Geometry: final body of the model. Coordinates: model frame, mm. A direction names the side the tool comes from. Coordinates: 2 decimals unless noted, no trailing zeros. Loops run counter-clockwise (first coordinate to the right, second up) from the corner with the lowest first, then second, coordinate; pieces in that order, holes last. Notation, with made-up numbers: (10, -34.75) - (43, -34.75) arc R18 cw to (43, -20.75) - close; hole circle Ø5 at (-32.5, 52). An arc over 180 degrees is marked (long way). Answer in a Markdown table with one row per item.
from build123d import *

# Parameters (mm, degrees)
SKETCH_R        = 14
SKETCH_R_2      = 2.5
PAD_DEPTH       = 16
SKETCH001_R     = 9
SKETCH001_R_2   = 2.5
PAD001_DEPTH    = 2.5
SKETCH002_R     = 3
SKETCH002_R_2   = 2.5
PAD002_DEPTH    = 2
CHAMFER_SIZE    = 0.5
CHAMFER001_SIZE = 1


with BuildPart() as part:
    # Sketch → Pad (new body)
    with BuildSketch(Plane.XY):
        with BuildLine():
            ThreePointArc((-14.073185, 9.536533), (-23.781107, 6.605863), (-16.975525, -0.911891))
            ThreePointArc((-16.975525, -0.911891), (-0.931565, -16.974457), (16.773787, -2.764066))
            Line((16.773787, -2.764066), (26.176697, -0.883484))
            ThreePointArc((26.176697, -0.883484), (30.883484, 6.176697), (23.823303, 10.883484))
            Line((23.823303, 10.883484), (14.420394, 9.002902))
            ThreePointArc((14.420394, 9.002902), (0.318322, 16.997019), (-14.073185, 9.536533))
        make_face()
        Circle(SKETCH_R, mode=Mode.SUBTRACT)
        with Locations((25, 5)):
            Circle(SKETCH_R_2, mode=Mode.SUBTRACT)
        with Locations((-18, 5)):
            Circle(SKETCH_R_2, mode=Mode.SUBTRACT)
    extrude(amount=PAD_DEPTH)

    # Sketch001 → Pad001 (join)
    with BuildSketch(Plane.XY.offset(16)):
        with BuildLine():
            ThreePointArc((-14.073185, 9.536533), (-23.781107, 6.605863), (-16.975525, -0.911891))
            ThreePointArc((-16.975525, -0.911891), (-0.931565, -16.974457), (16.773787, -2.764066))
            Line((16.773787, -2.764066), (26.176697, -0.883484))
            ThreePointArc((26.176697, -0.883484), (30.883484, 6.176697), (23.823303, 10.883484))
            Line((23.823303, 10.883484), (14.420394, 9.002902))
            ThreePointArc((14.420394, 9.002902), (0.318322, 16.997019), (-14.073185, 9.536533))
        make_face()
        Circle(SKETCH001_R, mode=Mode.SUBTRACT)
        with Locations((25, 5)):
            Circle(SKETCH001_R_2, mode=Mode.SUBTRACT)
        with Locations((-18, 5)):
            Circle(SKETCH001_R_2, mode=Mode.SUBTRACT)
    extrude(amount=PAD001_DEPTH)

    # Sketch002 → Pad002 (join)
    with BuildSketch(Plane.XY.offset(18)):
        with BuildLine():
            ThreePointArc((-14.073185, 9.536533), (-23.781107, 6.605863), (-16.975525, -0.911891))
            ThreePointArc((-16.975525, -0.911891), (-0.931565, -16.974457), (16.773787, -2.764066))
            Line((16.773787, -2.764066), (26.176697, -0.883484))
            ThreePointArc((26.176697, -0.883484), (30.883484, 6.176697), (23.823303, 10.883484))
            Line((23.823303, 10.883484), (14.420394, 9.002902))
            ThreePointArc((14.420394, 9.002902), (0.318322, 16.997019), (-14.073185, 9.536533))
        make_face()
        Circle(SKETCH002_R, mode=Mode.SUBTRACT)
        with Locations((25, 5)):
            Circle(SKETCH002_R_2, mode=Mode.SUBTRACT)
        with Locations((-18, 5)):
            Circle(SKETCH002_R_2, mode=Mode.SUBTRACT)
    extrude(amount=PAD002_DEPTH)

    # Chamfer
    chamfer_edges = [part.edges().sort_by_distance(p)[0] for p in [
        (-9, 0, 16),
    ]]
    chamfer(chamfer_edges, length=CHAMFER_SIZE)

    # Chamfer001
    chamfer001_edges = [part.edges().sort_by_distance(p)[0] for p in [
        (-3, 0, 18),
    ]]
    chamfer(chamfer001_edges, length=CHAMFER001_SIZE)


solid = part.part
(1) Cut plane B-B on y = 0. Output: boundary loops of the cut face in (x, z), then the cut area to 3 significant figures.
Verdict:
| item | result |
|---|---|
| outline | (-21.32, 0) - (-14, 0) - (-14, 16) - (-9.5, 16) - (-9, 16.5) - (-9, 18) - (-4, 18) - (-3, 19) - (-3, 20) - (-21.32, 20) - close; (3, 19) - (4, 18) - (9, 18) - (9, 16.5) - (9.5, 16) - (14, 16) - (14, 0) - (28.32, 0) - (28.32, 20) - (3, 20) - close |
| area | 495 mm² |
(2) Cut plane C-C on x = -18. Output: boundary loops of the cut face in (y, z).
Verdict:
| item | result |
|---|---|
| outline | (-1, 0) - (2.5, 0) - (2.5, 20) - (-1, 20) - close; (7.5, 0) - (11, 0) - (11, 20) - (7.5, 20) - close |
(3) Ray query, probe 1 along Y at (x, z) = (0, 17.35); probe 2 along X at (y, z) = (3, 16.75); probe 3 along Y at (x, z) = (0, 19.35). Return the intervals inside material, ascending.
Verdict:
| item | result |
|---|---|
| probe 1 | y = -17 to -9, 9 to 17 |
| probe 2 | x = -23.66 to -19.5, -16.5 to -8.49, 8.49 to 23.5, 26.5 to 30.66 |
| probe 3 | y = -17 to -3, 3 to 17 |
(4) Access query for faces 4 (the face through (-3, 0.1, 19.5)), 5 (the face through (-1.172, 8.923, 17.24)). Directions: +Z, -Z, +X, -X, +Y, -Y. A direction counts if a zero-diameter tool reaches every point of the face in a straight line with its end or side. Return the directions, or none.
Verdict:
| item | result |
|---|---|
| face 4 | +Z, -Z |
| face 5 | -Z |
(5) Cut plane A-A on x = 0. Output: boundary loops of the cut face in (y, z).
Verdict:
| item | result |
|---|---|
| outline | (-17, 0) - (-14, 0) - (-14, 16) - (-9.5, 16) - (-9, 16.5) - (-9, 18) - (-4, 18) - (-3, 19) - (-3, 20) - (-17, 20) - close; (3, 19) - (4, 18) - (9, 18) - (9, 16.5) - (9.5, 16) - (14, 16) - (14, 0) - (17, 0) - (17, 20) - (3, 20) - close |
(6) Pull-direction query (Y, two-part tool) for faces 1 (the face through (2, -4, 18)), 2 (the face through (19.188, 9.956, 9.86)), 3 (the face through (14, 5, 0)); classes: pulls with the +Y half, pulls with the -Y half, needs draft (parallel to the pull), parting line crosses it, or undercut.
Verdict:
| item | result |
|---|---|
| face 1 | undercut |
| face 2 | pulls with the +Y half |
| face 3 | needs draft |
(7) First-contact query: pin 1 Ø6 at (x, z) = (7, 2) entering from -Y; pin 2 Ø8.5 at (x, y) = (-0.5, -0.5) entering from -Z; pin 3 Ø10 at (x, z) = (-17.5, 11.5) entering from +Y. Flat tips, straight axial feed; report the tip coordinate or a pass-through.
Verdict:
| item | result |
|---|---|
| pin 1 | stops at y = -16.52 |
| pin 2 | stops at z = 18 |
| pin 3 | stops at y = 11.52 |
(8) Cut plane D-D on y = 5. State how many separate pieces and enclosed holes the cut face has, then the cut area to 3 significant figures.
Verdict:
| item | result |
|---|---|
| separate pieces | 3 |
| enclosed holes | 0 |
| area | 451 mm² |
